Geometry check sheet. Reference: the model listing, model coordinates, mm. A direction names the side the tool comes from. Coordinates: 2 decimals unless noted, no trailing zeros. Write each loop counter-clockwise with the first axis right and the second up, starting at its lowest first coordinate (ties: lowest second). Pieces come first, ordered by that corner, then holes.
Autodesk Inventor part; units mm, degrees
ref_plane "YZ Plane" through (0, 0, 0) normal (1, 0, 0) x (0, 1, 0)
ref_plane "XZ Plane" through (0, 0, 0) normal (0, 1, 0) x (-1, 0, 0)
ref_plane "XY Plane" through (0, 0, 0) normal (0, 0, 1) x (1, 0, 0)
sketch "Sketch1" plane through (0, 0, 0) normal (0, 1, 0) x (-1, 0, 0)
  line L0 (-127.7724, 127.5062) -> (122.2276, 127.5062)
  line L1 (122.2276, 127.5062) -> (122.2276, -122.4938)
  line L2 (122.2276, -122.4938) -> (-127.7724, -122.4938)
  line L3 (-127.7724, -122.4938) -> (-127.7724, 127.5062)
  line L4 (104.2276, -104.4938) -> (104.2276, 109.5062)
  line L5 (104.2276, -104.4938) -> (-109.7724, -104.4938)
  line L6 (-109.7724, -104.4938) -> (104.2276, -104.4938)
  line L7 (122.2276, 109.5062) -> (122.2276, 88.1062)
  line L8 (122.2276, 88.1062) -> (104.2276, 88.1062)
  line L9 (104.2276, 88.1062) -> (104.2276, 109.5062)
  line L10 (122.2276, 45.3062) -> (104.2276, 45.3062)
  line L11 (104.2276, 45.3062) -> (104.2276, 23.9062)
  line L12 (104.2276, 23.9062) -> (122.2276, 23.9062)
  line L13 (104.2276, -18.8938) -> (122.2276, -18.8938)
  line L14 (122.2276, -40.2938) -> (104.2276, -40.2938)
  line L15 (122.2276, -83.0938) -> (104.2276, -83.0938)
  line L16 (-127.7724, 127.5062) -> (-127.7724, 109.5062)
  line L17 (104.2276, 109.5062) -> (104.2276, 127.5062)
  line L18 (-127.7724, -83.0938) -> (-109.7724, -83.0938)
  line L19 (-127.7724, -40.2938) -> (-109.7724, -40.2938)
  line L20 (-109.7724, -18.8938) -> (-127.7724, -18.8938)
  line L21 (-109.7724, 23.9062) -> (-127.7724, 23.9062)
  line L22 (-127.7724, 45.3062) -> (-109.7724, 45.3062)
  line L23 (-127.7724, 88.1062) -> (-109.7724, 88.1062)
  line L24 (18.6276, -104.4938) -> (18.6276, -122.4938)
  line L25 (-24.1724, -104.4938) -> (-24.1724, -122.4938)
  line L26 (-45.5724, -122.4938) -> (-45.5724, -104.4938)
  line L27 (-88.3724, -122.4938) -> (-88.3724, -104.4938)
  line L28 (40.0276, -122.4938) -> (40.0276, -104.4938)
  line L29 (82.8276, -122.4938) -> (82.8276, -104.4938)
  line L30 (18.6276, 127.5062) -> (18.6276, 109.5062)
  line L31 (40.0276, 109.5062) -> (40.0276, 127.5062)
  line L32 (82.8276, 109.5062) -> (82.8276, 127.5062)
  line L33 (-45.5724, 109.5062) -> (-45.5724, 127.5062)
  line L34 (-88.3724, 109.5062) -> (-88.3724, 127.5062)
  line L35 (-24.1724, 127.5062) -> (-24.1724, 109.5062)
  line L36 (104.2276, 109.5062) -> (-109.7724, 109.5062)
  line L37 (-109.7724, 109.5062) -> (-109.7724, -104.4938)
  line L38 (-109.7724, 109.5062) -> (-127.7724, 109.5062)
  line L39 (-127.7724, 109.5062) -> (-127.7724, 127.5062)
  line L40 (-127.7724, 127.5062) -> (-109.7724, 127.5062)
  line L41 (-109.7724, 127.5062) -> (-109.7724, 109.5062)
  line L42 (-109.7724, -104.4938) -> (-127.7724, -104.4938)
  line L43 (-127.7724, -104.4938) -> (-127.7724, -122.4938)
  line L44 (-127.7724, -122.4938) -> (-109.7724, -122.4938)
  line L45 (-109.7724, -122.4938) -> (-109.7724, -104.4938)
  line L46 (104.2276, -104.4938) -> (122.2276, -104.4938)
  line L47 (122.2276, -104.4938) -> (122.2276, -122.4938)
  line L48 (122.2276, -122.4938) -> (104.2276, -122.4938)
  line L49 (104.2276, -122.4938) -> (104.2276, -104.4938)
  line L50 (104.2276, 109.5062) -> (122.2276, 109.5062)
  line L51 (122.2276, 109.5062) -> (122.2276, 127.5062)
  line L52 (122.2276, 127.5062) -> (104.2276, 127.5062)
  line L53 (104.2276, 127.5062) -> (104.2276, 109.5062)
  point P0 (0, 0)
  point P1 (-127.7724, -18.8938)
  point P2 (-109.7724, -104.4938)
  point P3 (-109.7724, -104.4938)
  dimension "d0" = 250
  dimension "d1" = 250
  dimension "d2" = 21.4
extrude "Plate1" add sketch "Sketch1" along normal blind 18 contours L38 L37 L23 L3 | L0 L33 L36 L34 | L36 L4 L5 L37 | L22 L37 L21 L3 | L0 L30 L36 L35 | L20 L37 L19 L3 | L0 L32 L36 L31 | L18 L37 L42 L3 | L50 L1 L8 L4 | L5 L26 L2 L27 | L10 L1 L12 L4 | L5 L24 L2 L25 | L13 L1 L14 L4 | L5 L29 L2 L28 | L15 L1 L46 L4
sketch "Sketch2" plane through (0, 0, 0) normal (0, -1, 0) x (1, 0, 0)
  line L0 (0, 0) -> (125, 0)
  line L1 (125, 0) -> (125, 125)
  line L2 (125, 125) -> (0, 125)
  line L3 (0, 125) -> (0, 0)
  line L4 (125, 125) -> (62.5, 125)
  line L5 (125, 62.5) -> (125, 125)
  circle A0 centre (62.5, 62.5) radius 44.45
  line L6 (25, 100) -> (100, 100)
  line L7 (100, 100) -> (100, 25)
  line L8 (100, 25) -> (25, 25)
  line L9 (25, 25) -> (25, 100)
  line L10 (25, 100) -> (100, 25) construction
  line L11 (100, 100) -> (25, 25) construction
  circle A1 centre (100, 100) radius 1.5
  circle A2 centre (100, 25) radius 1.5
  circle A3 centre (25, 25) radius 1.5
  circle A4 centre (25, 100) radius 1.5
  dimension "d4" = 125
  dimension "d5" = 125
  dimension "d6" = 88.9
  dimension "d7" = 75
  dimension "d8" = 75
  dimension "d9" = 3
  dimension "d10" = 3
  dimension "d11" = 3
  dimension "d12" = 3
extrude "Cut1" cut sketch "Sketch2" against normal blind 18 contours A0 L7 | L7 A0 L8 L9 L6 | L6 A0 | A1 L6 L7 | L7 L6 A1 | A0 L8 | A2 L8 L7 | L7 L8 A2 | L9 A0 | A4 L9 L6 | L6 L9 A4 | A3 L9 L8 | L8 L9 A3
ref_plane "Work Plane1" through (45.5724, 0, 2.5062) normal (0, 0, 1) x (1, 0, 0)
mirror "Mirror1" about plane through (45.5724, 0, 2.5062) normal (0, 0, 1) of "Cut1"
equation "\"d13\" = Thickness"
equation "\"d3\" = Thickness"
equation "\"BendRadius\" = Thickness"
equation "\"BendReliefWidth\" = Thickness"
equation "\"BendReliefDepth\" = 0.5 * Thickness"
equation "\"CornerReliefSize\" = 4 * Thickness"
equation "\"MinimumRemnant\" = 2 * Thickness"
equation "\"TransitionRadius\" = BendRadius"
equation "\"JacobiRadiusSize\" = BendRadius"
equation "\"GapSize\" = Thickness"
properties part number "4"
1. Sectioned sample at A-A, the plane z = 62.5. Record the boundary of the cut face in (x, y), and give its area (3 significant figures).
Computed values:
outline: (-104.23, 0) - (18.05, 0) - (18.05, 18) - (-104.23, 18) - close; (106.95, 0) - (109.77, 0) - (109.77, 18) - (106.95, 18) - close
area: 2,250 mm2
2. Thickness scan on line 1 along X through (y, z) = (6.5, -105); line 2 along Z through (x, y) = (62.5, 8.75); line 3 along X through (y, z) = (4.5, -96). Record the ranges inside material, lowest first.
Computed values:
line 1: x = -82.83 to -40.03, -18.63 to 24.17, 45.57 to 88.37
line 2: z = -122.49 to -101.94, -13.04 to 18.05, 106.95 to 127.51
line 3: x = -122.23 to 23.89, 26.11 to 40.31, 84.69 to 98.89, 101.11 to 127.77
3. Access from +Z, -Z, +X, -X, +Y, -Y to the whole of each face (thin tool, end or side, straight path). Record for faces 1 (the flat face through (108, 9, 109.506)), 2 (the flat face through (-29, 9, -104.494)), 3 (the flat face through (109.772, 9, -61)), 4 (the flat face through (-104.228, 9, -62)).
Computed values:
face 1: +Z, +X, +Y, -Y
face 2: -Z, +Y, -Y
face 3: +X, +Y, -Y
face 4: -X, +Y, -Y
4. Draft check along X on faces 5 (the flat face through (67, 9, -122.494)), 6 (the flat face through (88.372, 9, -114)), 7 (the flat face through (45.572, 9, -114)). Enter one of: released by +X, released by -X, zero draft, split by the parting line, or undercut.
Computed values:
face 5: zero draft
face 6: released by +X
face 7: undercut
5. Sectioned sample at C-C, the plane y = 7. Give the number of separate pieces and of enclosed holes in the cut face, and give its area (3 significant figures).
Computed values:
separate pieces: 1
enclosed holes: 10
area: 41,000 mm2
6. Sectioned sample at D-D, the plane z = 12.5. Record the boundary of the cut face in (x, y).
Computed values:
outline: (-104.23, 0) - (109.77, 0) - (109.77, 18) - (-104.23, 18) - close
7. Gauge pin test, flat ends, axial feed: pin 1 Ø5.5 at (x, y) = (120.5, 7) entering from +Z; pin 2 Ø9 at (y, z) = (13.5, -116) entering from +X; pin 3 Ø10 at (y, z) = (4.5, 55.5) entering from +X; pin 4 Ø1.8 at (x, z) = (25, -19.99) entering from +Y. Record the tip position at first contact, or that the pin passes through.
Computed values:
pin 1: stops at z = 109.51
pin 2: stops at x = 88.37
pin 3: stops at x = 109.77
pin 4: passes through
8. Sectioned sample at B-B, the plane x = 62.5. Record the boundary of the cut face in (y, z), and give its area (3 significant figures).
Computed values:
outline: (0, -122.49) - (18, -122.49) - (18, -101.94) - (0, -101.94) - close; (0, -13.04) - (18, -13.04) - (18, 18.05) - (0, 18.05) - close; (0, 106.95) - (18, 106.95) - (18, 127.51) - (0, 127.51) - close
area: 1,300 mm2
